Read the model definition and answer for the solid it produces. Units are mm, in the model's axes. A direction names the side the tool comes from. Give positions to 0.01 mm unless a question says otherwise; leave off trailing zeros. Order: outer loops, then holes, each group sorted by start corner. A loop starts at its lowest first (then second) coordinate and runs counter-clockwise, first axis right, second up. Notation, with made-up numbers: (41, 77.25) -> (59, 77.25) arc R23 ccw to (59, 86.25) -> close; hole circle Ø7 at (-39, 17). An arc over 180 degrees is marked (long way). Use one line per item in the form item = value.
```python
from build123d import *

# Parameters (mm, degrees)
SKETCH1_R           = 10
BOSS_EXTRUDE1_DEPTH = 10
SKETCH2_W           = 150
SKETCH2_H           = 150
BOSS_EXTRUDE2_DEPTH = 150
BOSS_EXTRUDE2_TAPER = 5
SKETCH3_R           = 20
CUT_EXTRUDE1_DEPTH  = 151.0000001
FILLET1_R           = 6


with BuildPart() as part:
    # Sketch1 → Boss-Extrude1 (new body)
    with BuildSketch(Plane(origin=(0, 0, 0), x_dir=(1, 0, 0), z_dir=(0, 1, 0))):
        with BuildLine():
            ThreePointArc((-120, -105), (-115.606601718, -115.606601718), (-105, -120))
            Line((-105, -120), (105, -120))
            ThreePointArc((105, -120), (115.606601718, -115.606601718), (120, -105))
            Line((120, -105), (120, 105))
            ThreePointArc((120, 105), (115.606601718, 115.606601718), (105, 120))
            Line((105, 120), (-105, 120))
            ThreePointArc((-105, 120), (-115.606601718, 115.606601718), (-120, 105))
            Line((-120, 105), (-120, -105))
        make_face()
        with Locations((-100, -100)):
            Circle(SKETCH1_R, mode=Mode.SUBTRACT)
        with Locations((100, -100)):
            Circle(SKETCH1_R, mode=Mode.SUBTRACT)
        with Locations((-100, 100)):
            Circle(SKETCH1_R, mode=Mode.SUBTRACT)
        with Locations((100, 100)):
            Circle(SKETCH1_R, mode=Mode.SUBTRACT)
    extrude(amount=BOSS_EXTRUDE1_DEPTH)

    # Sketch2 → Boss-Extrude2 (add)
    with BuildSketch(Plane(origin=(0, 0, 0), x_dir=(1, 0, 0), z_dir=(0, 1, 0))):
        Rectangle(SKETCH2_W, SKETCH2_H)
    extrude(amount=BOSS_EXTRUDE2_DEPTH, taper=BOSS_EXTRUDE2_TAPER)

    # Sketch3 → Cut-Extrude1 (cut, through all)
    with BuildSketch(Plane(origin=(0, 0, 0), x_dir=(1, 0, 0), z_dir=(0, 1, 0))):
        Circle(SKETCH3_R)
    extrude(amount=CUT_EXTRUDE1_DEPTH, mode=Mode.SUBTRACT)

    # Fillet1
    fillet1_edges = [part.edges().sort_by_distance(p)[0] for p in [
        (-120, 10, 0),
        (-115.606601718, 10, 115.606601718),
        (0, 10, 120),
        (115.606601718, 10, 115.606601718),
        (120, 10, 0),
        (115.606601718, 10, -115.606601718),
        (0, 10, -120),
        (74.125113365, 10, 0),
        (0, 10, -74.125113365),
        (-74.125113365, 10, 0),
        (0, 10, 74.125113365),
        (68.000906918, 80, 68.000906918),
        (68.000906918, 80, -68.000906918),
        (-68.000906918, 80, -68.000906918),
        (-68.000906918, 80, 68.000906918),
        (61.876700471, 150, 0),
        (0, 150, -61.876700471),
        (-61.876700471, 150, 0),
        (0, 150, 61.876700471),
        (-115.606601718, 10, -115.606601718),
    ]]
    fillet(fillet1_edges, radius=FILLET1_R)


solid = part.part
```
Item 1: The part is cut by section B-B on z = -100. Give the vertices of the cut face in (x, y), and give its area (3 significant figures).
Checks:
outline = (-120, 0) -> (-110, 0) -> (-110, 10) -> (-114, 10) arc R6 ccw to (-120, 4) -> close; (-90, 0) -> (90, 0) -> (90, 10) -> (-90, 10) -> close; (110, 0) -> (120, 0) -> (120, 4) arc R6 ccw to (114, 10) -> (110, 10) -> close
area = 1,980 mm²
Item 2: Given pin 1 Ø8 at (y, z) = (49.5, 57.5) entering from +X; pin 2 Ø1 at (x, y) = (63, 102) entering from -Z; pin 3 Ø1.5 at (y, z) = (41.5, -29.5) entering from -X, each flat-ended and moving along its own axis, determine where each tip first touches the part or whether it passes through.
Checks:
pin_1 = 71.02
pin_2 = -65.58
pin_3 = -71.43
Item 3: Straight lines are drawn through the part: L1, parallel to X at y = 5, z = -100; L2, parallel to Y at x = 44, z = -99; L3, parallel to X at y = 80, z = 0. For each, find the intervals that lie inside material, in ascending order. Write a range as from..to.
Checks:
L1 = -119.92..-110, -90..90, 110..119.92
L2 = 0..10
L3 = -68..-20, 20..68
Item 4: Which of the six approach directions +Z, -Z, +X, -X, +Y, -Y give full straight-line access (tool end or side, diameter ignored) to faces 4 (the cylindrical face through (-101.302, 4.93, -109.915)), 5 (the flat face through (-103, 10, -2))?
Checks:
face_4 = +Y, -Y
face_5 = +Y
Item 5: The part is cut by section A-A on x = 100. Give the vertices of the cut face in (y, z), and give its area (3 significant figures).
Checks:
outline = (0, -120) -> (4, -120) arc R6 ccw to (10, -114) -> (10, -110) -> (0, -110) -> close; (0, -90) -> (10, -90) -> (10, 90) -> (0, 90) -> close; (0, 110) -> (10, 110) -> (10, 114) arc R6 ccw to (4, 120) -> (0, 120) -> close
area = 1,980 mm²
Item 6: Determine the mould class of faces 1 (the cylindrical face through (-115.49, 1.97, -115.72)), 2 (the cylindrical face through (115.72, 1.97, -115.49)), 3 (the cylindrical face through (-107.37, 4.93, 93.24)) for opening direction X: +X half, -X half, draft (parallel to the pull), parting line (faces both ways), or undercut.
Checks:
face_1 = -X half
face_2 = +X half
face_3 = undercut
